For this review, use the dimensioned drawing (mm, ordinates from the lowest corner) and the shaded views. Give positions to 0.01 mm unless a question says otherwise; leave off trailing zeros. Write each question's results on one line, items separated by ' | '. Start each with the question number.
Q1. Insertion check: pin 1 Ø2 at (y, z) = (1, 88) entering from -X; pin 2 Ø2 at (y, z) = (5, 60.5) entering from +X (1 decimal); pin 3 Ø2 at (y, z) = (4, 32.5) entering from +X (1 decimal). Each pin has a flat end and moves straight along its axis. Give the tip position at first contact, or say it passes through.
Q2. Wall thickness on L1, parallel to X at y = 4.75, z = 44.45; L2, parallel to X at y = 1.5, z = 25.4 (1 decimal); L3, parallel to X at y = 4.5, z = 142 (1 decimal): over which ranges is each line inside the solid? List them lowest first. Write a range as [from, to].
Q3. We need section A-A (y = 5.25). Give the number of separate pieces and of enclosed holes in the cut face, plus the area to 3 significant figures.
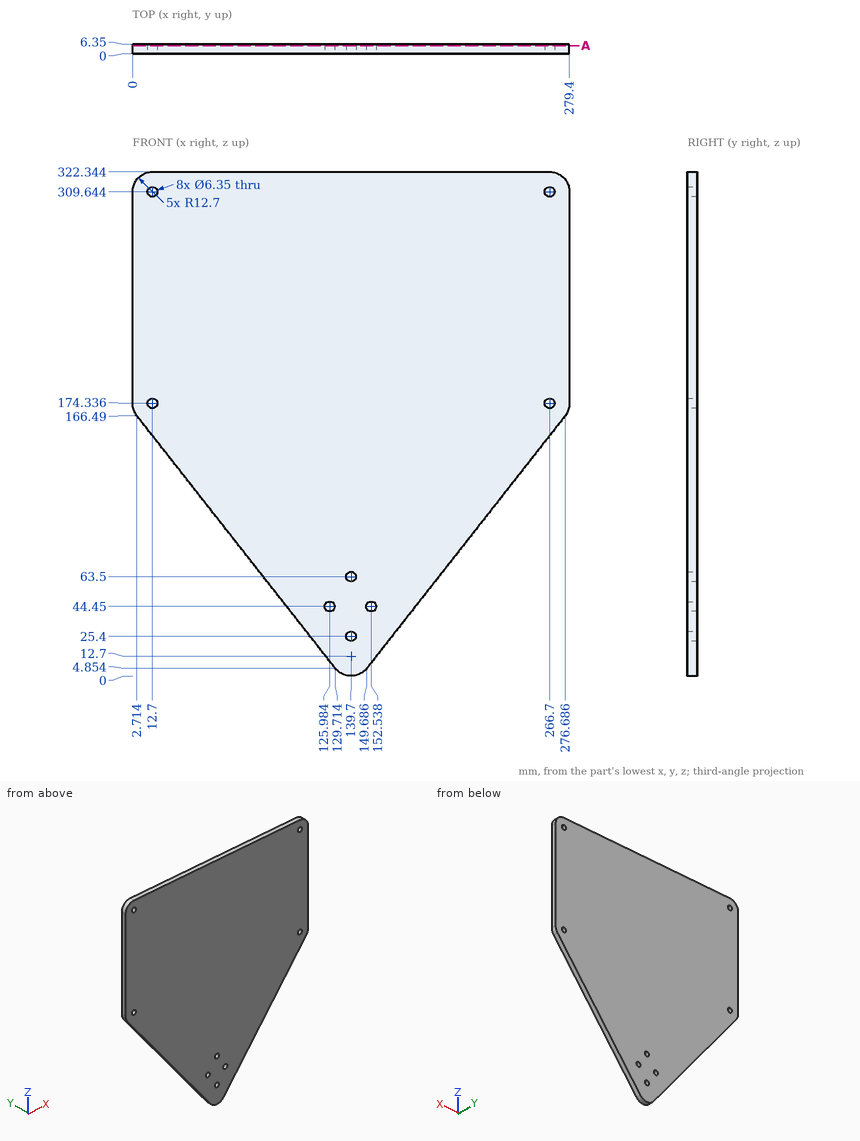
Output:
1) pin 1: x = 63.6 | pin 2: x = 194.2 | pin 3: x = 172.2
2) L1: [98.6, 122.81], [129.16, 149.36], [155.71, 180.8] | L2: [113.6, 136.5], [142.9, 165.8] | L3: [22, 257.4]
3) separate pieces: 1 | enclosed holes: 8 | area: 67,000 mm2
